Geometry: final body of the model. Coordinates: model frame, mm. A direction names the side the tool comes from. Give positions to 0.01 mm unless a question says otherwise; leave off trailing zeros. Write each loop counter-clockwise with the first axis right and the second up, starting at its lowest first coordinate (ties: lowest second). Pieces come first, ordered by that corner, then holes. Notation, with made-up numbers: M 84,27 L 122,27 A19 ccw 122,50 Z; hole C 4.5,62.25 d4. An arc over 180 degrees is marked long. One line per question, with ' | ' between items.
from build123d import *

# Parameters (mm, degrees)
F0_R     = 4.826
F1_DEPTH = 22.86
F2_R     = 6.35
F2_R_2   = 4.826
F3_DEPTH = 6.35
F4_DEPTH = 6.35


# Not quite as in the source:
# - a feature names something its author has since deleted; it is built from what else it names


with BuildPart() as f1:
    # F0 (on Top) → F1 (new body)
    with BuildSketch(Plane.XY):
        Circle(F0_R)
    extrude(amount=F1_DEPTH)

    # F2 (on face) → F3 (join)
    with BuildSketch(Plane.XY.offset(22.86)):
        Circle(F2_R)
        Circle(F2_R_2, mode=Mode.SUBTRACT)
    extrude(amount=F3_DEPTH)

    # F4 (add): a face of the model
    f4_faces = [f1.faces().sort_by_distance(p)[0] for p in [
        (0, 0, 22.86),
    ]]
    extrude(f4_faces, amount=F4_DEPTH)


solid = f1.part
(1) First-contact query: P1, Ø5, axis at x = -4, y = 0.5, coming from the -Z side; P2, Ø5, axis at y = -0.5, z = 14, coming from the -X side; P3, Ø2, axis at y = 4, z = 9.5, coming from the -X side. Flat tips, straight axial feed; report the tip coordinate or a pass-through.
Working result:
P1: stops at z = 0 | P2: stops at x = -4.83 | P3: stops at x = -3.78
(2) Set-up query: faces 1 (the face through (-1, 5, 22.86)), 2 (the face through (0, 0, 0)). Return all of +Z, -Z, +X, -X, +Y, -Y with unobstructed straight access to the full face (end or side cutting, diameter ignored); none if empty.
Working result:
face 1: -Z | face 2: -Z, +X, -X, +Y, -Y
(3) Cut plane C-C, the plane z = 2.5. Return loops of the section in (x, y), then the cut area to 3 significant figures.
Working result:
outline: C 0,0 d9.65 | area: 73.2 mm^2
(4) Cut plane A-A, the plane x = 0. Return loops of the section in (y, z), then the cut area to 3 significant figures.
Working result:
outline: M -6.35,22.86 L -4.83,22.86 L -4.83,0 L 4.83,0 L 4.83,22.86 L 6.35,22.86 L 6.35,29.21 L -6.35,29.21 Z | area: 301 mm^2
(5) Cut plane D-D, the plane z = 24. Return loops of the section in (x, y).
Working result:
outline: C 0,0 d12.7
(6) Material intervals for L1, parallel to Z at x = 6, y = -0.5; L2, parallel to X at y = -3.5, z = 19.75; L3, parallel to X at y = -4.5, z = 26.25, sorted ascending. Write a range as [from, to].
Working result:
L1: z = [22.86, 29.21] | L2: x = [-3.32, 3.32] | L3: x = [-4.48, 4.48]
